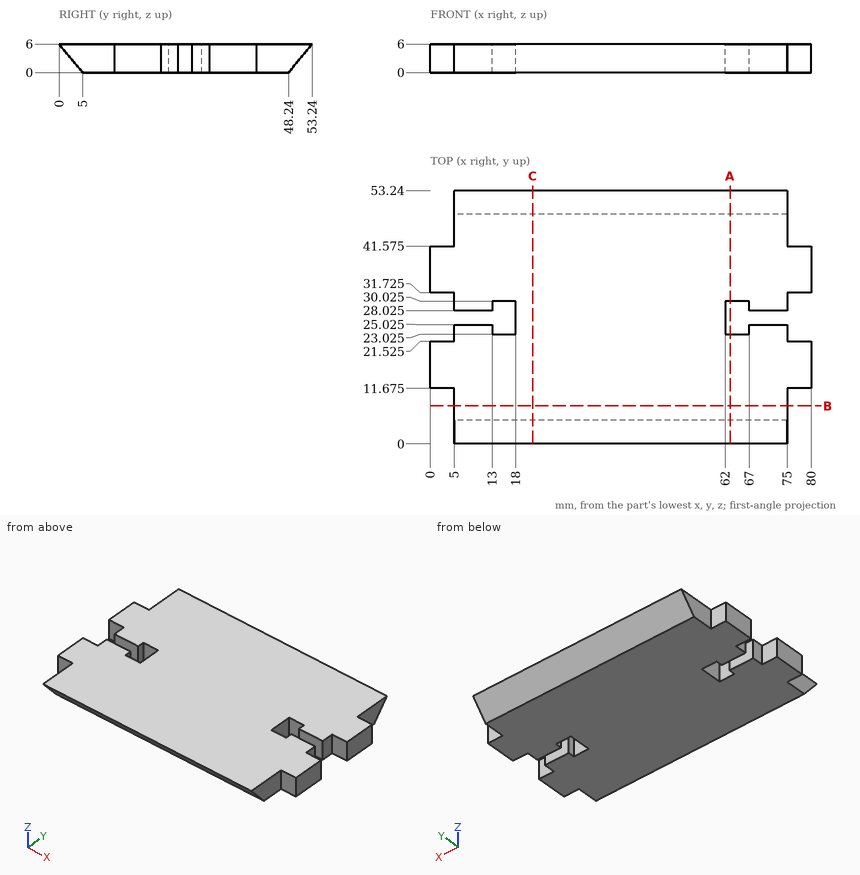
Drawing for the job (mm, zero at the part's lowest x, y, z). Round coordinates to 2 decimals unless told otherwise and drop trailing zeros. Write each loop counter-clockwise with the first axis right and the second up, starting at its lowest first coordinate (ties: lowest second). Pieces come first, ordered by that corner, then holes. Notation, with made-up numbers: (-22, 37) - (0, 37) arc R25 ccw to (0, 55) - close; hole circle Ø10 at (81, 62.25). An arc over 180 degrees is marked (long way). Return JSON: item names as keys, results as strings. Group by question number.
Item 1: Band-saw the part on A-A on x = 63. List the corners of the cut face in (y, z) (3 decimals).
Item 2: Band-saw the part on B-B on y = 8. List the corners of the cut face in (x, z), plus the area to 3 significant figures.
Item 3: Band-saw the part on C-C on x = 21.5. List the corners of the cut face in (y, z), plus the area to 3 significant figures.
Item 4: Flat gauge pins, fed straight in: pin 1 Ø2.5 at (x, z) = (2, 2.5) entering from +Y (3 decimals); pin 2 Ø1 at (y, z) = (24.5, 5.5) entering from +X; pin 3 Ø1.1 at (y, z) = (30.5, 3.5) entering from -X; pin 4 Ø1 at (x, y) = (29, 39) entering from -Z. Where does each tip first touch, or does it go through?
Item 5: Probe probe 1 along X at (y, z) = (24, 5); probe 2 along Y at (x, z) = (75.5, 3.2) (3 decimals); probe 3 along Y at (x, z) = (66.5, 4.8) (3 decimals). List the from-to ranges inside material, lowest first.
Resolved:
{
 "1": {"outline": "(0, 6) - (5, 0) - (23.025, 0) - (23.025, 6) - close; (30.025, 0) - (48.24, 0) - (53.24, 6) - (30.025, 6) - close"},
 "2": {"outline": "(5, 0) - (75, 0) - (75, 6) - (5, 6) - close", "area": "420 mm²"},
 "3": {"outline": "(0, 6) - (5, 0) - (48.24, 0) - (53.24, 6) - close", "area": "289 mm²"},
 "4": {"pin 1": "stops at y = 41.575", "pin 2": "stops at x = 75", "pin 3": "stops at x = 5", "pin 4": "stops at z = 0"},
 "5": {"probe 1": "x = 5 to 13, 18 to 62, 67 to 75", "probe 2": "y = 11.675 to 21.525, 31.725 to 41.575", "probe 3": "y = 1 to 23.025, 30.025 to 52.24"}
}
